Drawing for the job (mm, zero at the part's lowest x, y, z). A direction names the side the tool comes from. Give positions to 0.01 mm unless a question says otherwise; leave off trailing zeros. Loops run counter-clockwise (first coordinate to the right, second up) from the corner with the lowest first, then second, coordinate; pieces in that order, holes last.
1) Two-plate mould, pull along Y, no slides. Class the marked faces 3, 4 and 5: +Y half, -Y half, draft (parallel to the pull), parting line (faces both ways), or undercut.
2) Band-saw the part on B-B on z = 16.5. List the corners of the cut face in (x, y).
3) Flat gauge pins, fed straight in: P1, Ø6, axis at y = 20.5, z = 10.5, coming from the +X side; P2, Ø1.5, axis at y = 40.5, z = 18.5, coming from the +X side; P3, Ø10, axis at x = 9, y = 14.5, coming from the +Z side; P4, Ø1.5, axis at x = 19, z = 16.5, coming from the +Y side. Where does each tip first touch, or does it go through?
4) 3-axis set-ups, long thin cutter, end or side, ignore diameter. For the marked faces 1 and 2: which of +Z, -Z, +X, -X, +Y, -Y reach the whole face in a straight line?
5) Band-saw the part on A-A on x = 11.5. List the corners of the cut face in (y, z), then the cut area to 3 significant figures.
6) Band-saw the part on C-C on y = 20. List the corners of the cut face in (x, z).
7) Wall check: line 1 (Y direction, x = 8.25, z = 25.25); line 2 (X direction, y = 29.5, z = 7); line 3 (X direction, y = 40, z = 20). Give the ranges that are in metal, low to high.
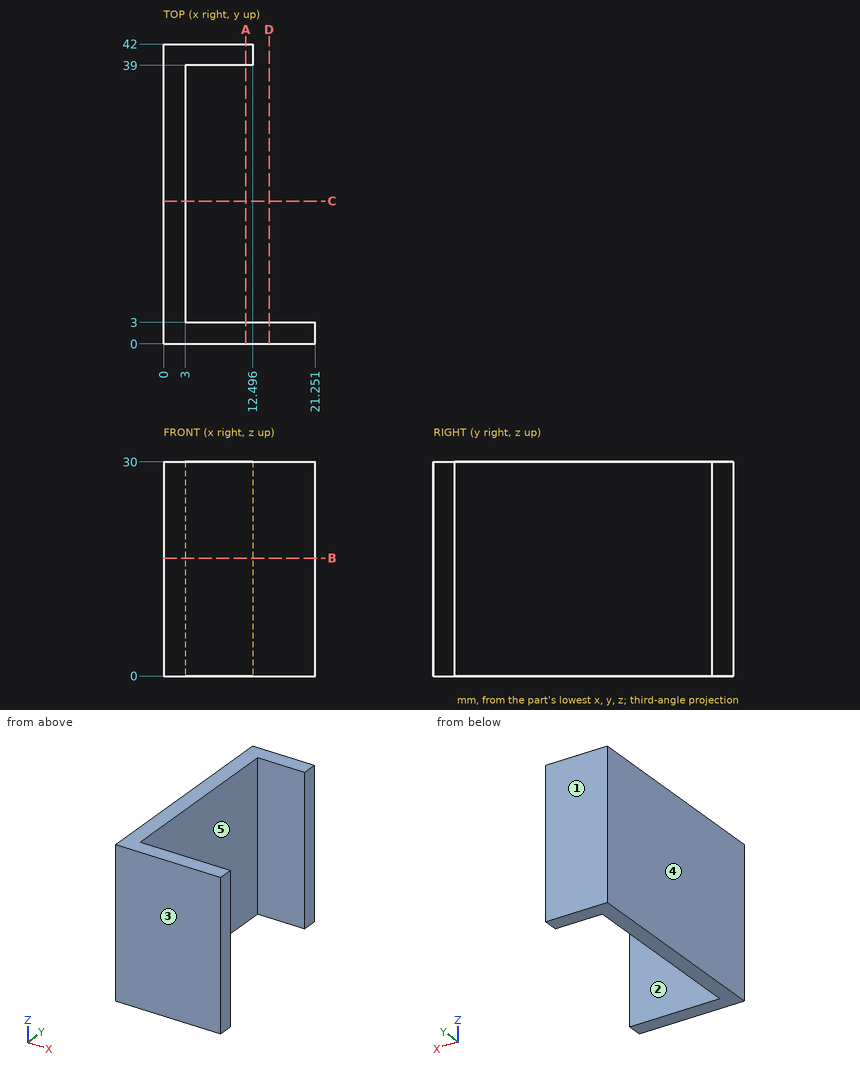
Findings below:
1. face 3: -Y half
1. face 4: draft
1. face 5: undercut
2. outline: (0, 0) - (21.25, 0) - (21.25, 3) - (3, 3) - (3, 39) - (12.5, 39) - (12.5, 42) - (0, 42) - close
3. P1: stops at x = 3
3. P2: stops at x = 12.5
3. P3: passes through
3. P4: stops at y = 3
4. face 1: +Z, -Z, +X, -X, +Y
4. face 2: +Z, -Z, +X
5. outline: (0, 0) - (3, 0) - (3, 30) - (0, 30) - close; (39, 0) - (42, 0) - (42, 30) - (39, 30) - close
5. area: 180 mm2
6. outline: (0, 0) - (3, 0) - (3, 30) - (0, 30) - close
7. line 1: y = 0 to 3, 39 to 42
7. line 2: x = 0 to 3
7. line 3: x = 0 to 12.5
